Geometry check sheet. Reference: the model listing, model coordinates, mm. A direction names the side the tool comes from. Coordinates: 2 decimals unless noted, no trailing zeros. Write each loop counter-clockwise with the first axis right and the second up, starting at its lowest first coordinate (ties: lowest second). Pieces come first, ordered by that corner, then holes.
from build123d import *

# Parameters (mm, degrees)
SKETCH1_W           = 5
SKETCH1_H           = 55
BOSS_EXTRUDE1_DEPTH = 15
FILLET1_R           = 5
SKETCH2_W           = 3
SKETCH2_H           = 10
CUT_EXTRUDE1_DEPTH  = 5
SKETCH3_R           = 3.75
BOSS_EXTRUDE2_DEPTH = 12
SKETCH4_R           = 1.75
BOSS_EXTRUDE3_DEPTH = 6


with BuildPart() as part:
    # Sketch1 → Boss-Extrude1 (new body)
    with BuildSketch(Plane(origin=(0, 0, 0), x_dir=(1, 0, 0), z_dir=(0, 1, 0))):
        with Locations((-59.380536913, 1.290268456)):
            Rectangle(SKETCH1_W, SKETCH1_H)
    extrude(amount=BOSS_EXTRUDE1_DEPTH)

    # Fillet1
    fillet1_edges = [part.edges().sort_by_distance(p)[0] for p in [
        (-59.380536913, 15, 26.209731544),
        (-59.380536913, 0, 26.209731544),
    ]]
    fillet(fillet1_edges, radius=FILLET1_R)

    # Sketch2 → Cut-Extrude1 (cut)
    with BuildSketch(Plane.ZY.offset(61.880536913)):
        with Locations((-25.290268456, 7.5)):
            Rectangle(SKETCH2_W, SKETCH2_H)
    extrude(amount=-CUT_EXTRUDE1_DEPTH, mode=Mode.SUBTRACT)

    # Sketch3 → Boss-Extrude2 (add)
    with BuildSketch(Plane.ZY.offset(61.880536913)):
        with Locations((21.209731544, 7.5)):
            Circle(SKETCH3_R)
    extrude(amount=BOSS_EXTRUDE2_DEPTH)

    # Sketch4 → Boss-Extrude3 (add)
    with BuildSketch(Plane.ZY.offset(73.880536913)):
        with Locations((21.209731544, 7.5)):
            Circle(SKETCH4_R)
    extrude(amount=BOSS_EXTRUDE3_DEPTH)


solid = part.part
1. Sectioned sample at C-C, the plane z = 0.5. Record the boundary of the cut face in (x, y).
Computed values:
outline: (-61.88, 0) - (-56.88, 0) - (-56.88, 15) - (-61.88, 15) - close
2. Sectioned sample at D-D, the plane x = -64.25. Record the boundary of the cut face in (y, z).
Computed values:
outline: circle Ø7.5 at (7.5, 21.21)
3. Thickness scan on line 1 along X through (y, z) = (14.25, -5.5); line 2 along Z through (x, y) = (-61.75, 3); line 3 along Z through (x, y) = (-60.75, 11). Record the ranges inside material, lowest first.
Computed values:
line 1: x = -61.88 to -56.88
line 2: z = -28.79 to -26.79, -23.79 to 25.79
line 3: z = -28.79 to -26.79, -23.79 to 26.11
4. Gauge pin test, flat ends, axial feed: pin 1 Ø5 at (x, y) = (-72, 3) entering from +Z; pin 2 Ø7.5 at (y, z) = (11, 3) entering from -X; pin 3 Ø6 at (x, y) = (-74, 13.5) entering from -Z. Record the tip position at first contact, or that the pin passes through.
Computed values:
pin 1: stops at z = 24.38
pin 2: stops at x = -61.88
pin 3: stops at z = 18.96
5. Sectioned sample at B-B, the plane x = -60.75. Record the boundary of the cut face in (y, z), and give its area (3 significant figures).
Computed values:
outline: (0, -28.79) - (15, -28.79) - (15, 21.21) arc R5 ccw to (10, 26.21) - (5, 26.21) arc R5 ccw to (0, 21.21) - close; hole (2.5, -26.79) - (12.5, -26.79) - (12.5, -23.79) - (2.5, -23.79) - close
area: 784 mm2
6. Access from +Z, -Z, +X, -X, +Y, -Y to the whole of each face (thin tool, end or side, straight path). Record for faces 1 (the flat face through (-73.881, 6, 20)), 2 (the flat face through (-59, 7, -23.79)), 3 (the flat face through (-59, 0, -4)).
Computed values:
face 1: -X
face 2: +X, -X
face 3: +Z, -Z, +X, -X, -Y
7. Draft check along Z on faces 4 (the flat face through (-79.881, 8, 21)), 5 (the flat face through (-59, 7, -26.79)), 6 (the cylindrical face through (-67.797, 8.626, 24.787)). Enter one of: released by +Z, released by -Z, zero draft, split by the parting line, or undercut.
Computed values:
face 4: zero draft
face 5: undercut
face 6: split by the parting line
8. Sectioned sample at A-A, the plane y = 7.5. Record the boundary of the cut face in (x, z).
Computed values:
outline: (-79.88, 19.46) - (-73.88, 19.46) - (-73.88, 17.46) - (-61.88, 17.46) - (-61.88, -23.79) - (-56.88, -23.79) - (-56.88, 26.21) - (-61.88, 26.21) - (-61.88, 24.96) - (-73.88, 24.96) - (-73.88, 22.96) - (-79.88, 22.96) - close; (-61.88, -28.79) - (-56.88, -28.79) - (-56.88, -26.79) - (-61.88, -26.79) - close
